```python
from build123d import *

# Parameters (mm, degrees)
SALIENTE_EXTRUIR1_DEPTH = 10


with BuildPart() as part:
    # Croquis1 → Saliente-Extruir1 (new body)
    with BuildSketch(Plane.XY):
        with BuildLine():
            Line((0, 0), (0, 40))
            Line((0, 40), (15, 55))
            Line((15, 55), (71.937253933, 55))
            Line((71.937253933, 55), (79.937253933, 49))
            Line((79.937253933, 49), (79.937253933, 15))
            ThreePointArc((79.937253933, 15), (71.436270633, 7.015701926), (64, 16))
            ThreePointArc((64, 16), (62.062746067, 22.291502622), (56.062746067, 25))
            Line((56.062746067, 25), (35, 25))
            ThreePointArc((35, 25), (24.393398282, 20.606601718), (20, 10))
            Line((20, 10), (20, 0))
            ThreePointArc((20, 0), (10, -10), (0, 0))
        make_face()
        Polygon((20, 44), (23, 47), (42, 47), (45, 44), (45, 35), (42, 32), (23, 32), (20, 35), align=None, mode=Mode.SUBTRACT)
    extrude(amount=SALIENTE_EXTRUIR1_DEPTH)


solid = part.part
```
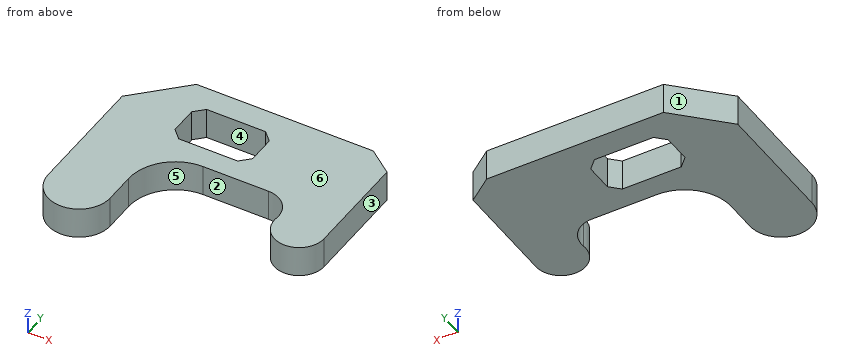
Read the model definition and answer for the solid it produces. Units are mm, in the model's axes. Face numbers are marked on the shaded views. A direction names the side the tool comes from. Coordinates: 2 decimals unless noted, no trailing zeros. Write each loop counter-clockwise with the first axis right and the second up, starting at its lowest first coordinate (ties: lowest second). Pieces come first, ordered by that corner, then holes. Notation, with made-up numbers: (-39.75, 30) -> (-1.75, 30) arc R20 ccw to (-1.75, 41) -> close; hole circle Ø6 at (66, 62). An arc over 180 degrees is marked (long way). Return JSON: item names as keys, results as strings.
1. Each of these flat-tipped pins is pushed along its axis until it touches: P1, Ø5, axis at x = 34, z = 3.5, coming from the -Y side; P2, Ø3, axis at x = 44.5, z = 4.5, coming from the -Y side; P3, Ø2, axis at y = -0.5, z = 4.5, coming from the +X side. Where does it stop, or does it pass through?
Found:
{"P1": "y = 24.59", "P2": "y = 25", "P3": "x = 20"}
2. A cutting plane is placed at A-A (z = 8.75). Determine the outline of the cut face in (x, y).
Found:
{"outline": "(0, 0) arc R10 ccw to (20, 0) -> (20, 10) arc R15 cw to (35, 25) -> (56.06, 25) arc R8 cw to (64, 16) arc R8 ccw (long way) to (79.94, 15) -> (79.94, 49) -> (71.94, 55) -> (15, 55) -> (0, 40) -> close; hole (20, 35) -> (23, 32) -> (42, 32) -> (45, 35) -> (45, 44) -> (42, 47) -> (23, 47) -> (20, 44) -> close"}
3. A tool of negligible diameter and unlimited length cuts with its end or side. For the marked faces 4, 5 and 6, from which of +Z, -Z, +X, -X, +Y, -Y can it reach the whole face along a straight path? Write none if from no direction.
Found:
{"face 4": "+Z, -Z", "face 5": "+Z, -Z, -Y", "face 6": "+Z, +X, -X, +Y, -Y"}
4. A cutting plane is placed at C-C (y = 20). Determine the outline of the cut face in (x, z).
Found:
{"outline": "(0, 0) -> (23.82, 0) -> (23.82, 10) -> (0, 10) -> close; (63.48, 0) -> (79.94, 0) -> (79.94, 10) -> (63.48, 10) -> close"}
5. A cutting plane is placed at B-B (y = 13.5). Determine the outline of the cut face in (x, z), and give its area (3 significant figures).
Found:
{"outline": "(0, 0) -> (20.41, 0) -> (20.41, 10) -> (0, 10) -> close; (64.08, 0) -> (79.8, 0) -> (79.8, 10) -> (64.08, 10) -> close", "area": "361 mm2"}
6. Find the intervals of material crossed by line 1 along X through (y, z) = (36, 4.5); line 2 along Y through (x, z) = (39, 4); line 3 along Y through (x, z) = (22, 2.5), in increasing order. Write a range as from..to.
Found:
{"line 1": "0..20, 45..79.94", "line 2": "25..32, 47..55", "line 3": "17.48..33, 46..55"}
7. A cutting plane is placed at D-D (x = 54). Determine the outline of the cut face in (y, z).
Found:
{"outline": "(25, 0) -> (55, 0) -> (55, 10) -> (25, 10) -> close"}
8. Determine the mould class of the marked faces 1, 2 and 3 for opening direction X: pulls with the +X half, pulls with the -X half, needs draft (parallel to the pull), parting line crosses it, or undercut.
Found:
{"face 1": "pulls with the -X half", "face 2": "undercut", "face 3": "pulls with the +X half"}
